Here's the drawing with two shaded views (mm, measured from the low corner). I have some questions. A direction names the side the tool comes from. Round coordinates to 2 decimals unless told otherwise and drop trailing zeros. Order: outer loops, then holes, each group sorted by start corner. A loop starts at its lowest first (then second) coordinate and runs counter-clockwise, first axis right, second up. Notation, with made-up numbers: (24, -35) -> (49, -35) arc R20 cw to (49, -9) -> close; hole circle Ø6 at (6, 25). An arc over 180 degrees is marked (long way). Answer in a Markdown table with one row per item.
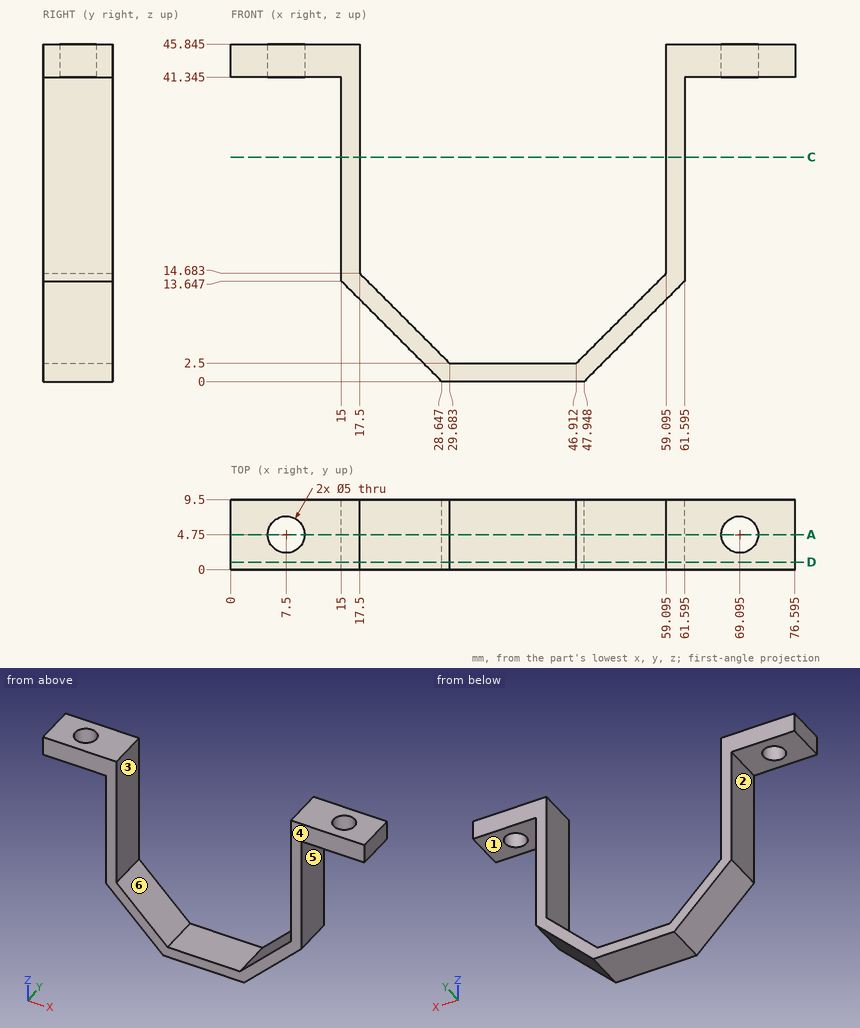
1. Suppose I cut it at A-A on y = 4.75. Write out the boundary of the cut face in (x, z) (1 decimal).
Numbers:
| item | result |
|---|---|
| outline | (0, 41.3) -> (5, 41.3) -> (5, 45.8) -> (0, 45.8) -> close; (10, 41.3) -> (15, 41.3) -> (15, 13.6) -> (28.6, 0) -> (47.9, 0) -> (61.6, 13.6) -> (61.6, 41.3) -> (66.6, 41.3) -> (66.6, 45.8) -> (59.1, 45.8) -> (59.1, 14.7) -> (46.9, 2.5) -> (29.7, 2.5) -> (17.5, 14.7) -> (17.5, 45.8) -> (10, 45.8) -> close; (71.6, 41.3) -> (76.6, 41.3) -> (76.6, 45.8) -> (71.6, 45.8) -> close |
2. For the marked faces 1, 2 and 3, which set-ups out of +Z, -Z, +X, -X, +Y, -Y let a thin tool reach every point of the face, with its end or its side?
Numbers:
| item | result |
|---|---|
| face 1 | -Z, +X, +Y, -Y |
| face 2 | -Z, -X, +Y, -Y |
| face 3 | +Z, +Y, -Y |
3. Suppose I cut it at D-D on y = 1. Write out the boundary of the cut face in (x, z) (1 decimal).
Numbers:
| item | result |
|---|---|
| outline | (0, 41.3) -> (15, 41.3) -> (15, 13.6) -> (28.6, 0) -> (47.9, 0) -> (61.6, 13.6) -> (61.6, 41.3) -> (76.6, 41.3) -> (76.6, 45.8) -> (59.1, 45.8) -> (59.1, 14.7) -> (46.9, 2.5) -> (29.7, 2.5) -> (17.5, 14.7) -> (17.5, 45.8) -> (0, 45.8) -> close |
4. We'd pull the mould along X, two halves only. Please class the marked faces 4, 5 and 6: released by +X, released by -X, zero draft, split by the parting line, or undercut.
Numbers:
| item | result |
|---|---|
| face 4 | zero draft |
| face 5 | released by +X |
| face 6 | undercut |
5. Please list where these lines run through material, in increasing order: line 1 along Z through (x, y) = (30, 2.5); line 2 along Z through (x, y) = (8, 7.5) (1 decimal); line 3 along X through (y, z) = (6.5, 27) (1 decimal).
Numbers:
| item | result |
|---|---|
| line 1 | z = 0 to 2.5 |
| line 2 | z = 41.3 to 45.8 |
| line 3 | x = 15 to 17.5, 59.1 to 61.6 |
6. For pin 1 Ø5 at (x, y) = (40, 3.5) entering from +Z; pin 2 Ø2 at (x, y) = (22, 4.5) entering from -Z; pin 3 Ø3 at (x, y) = (6, 4.5) entering from -Z (3 decimals); pin 4 Ø1 at (x, z) = (58.5, 34) entering from -Y, each with a flat end and sliding along its axis, tell me the tip position at first contact or that it passes through.
Numbers:
| item | result |
|---|---|
| pin 1 | stops at z = 2.5 |
| pin 2 | stops at z = 5.65 |
| pin 3 | stops at z = 41.345 |
| pin 4 | passes through |
7. Suppose I cut it at C-C on z = 30.5. Write out the boundary of the cut face in (x, y) (1 decimal), then the cut area to 3 significant figures.
Numbers:
| item | result |
|---|---|
| outline | (15, 0) -> (17.5, 0) -> (17.5, 9.5) -> (15, 9.5) -> close; (59.1, 0) -> (61.6, 0) -> (61.6, 9.5) -> (59.1, 9.5) -> close |
| area | 47.5 mm2 |
